Print and shaded views of the part. All mm, measured from the part's lowest x, y and z. A direction names the side the tool comes from. Give positions to 0.01 mm unless a question says otherwise; leave off trailing zeros. Loops run counter-clockwise (first coordinate to the right, second up) from the corner with the lowest first, then second, coordinate; pieces in that order, holes last. Notation, with made-up numbers: M 29,-16 L 52,-16 A33 ccw 52,18 Z; hole C -18,56 d1. An arc over 180 degrees is marked long. Answer in a Markdown table with one row per item.
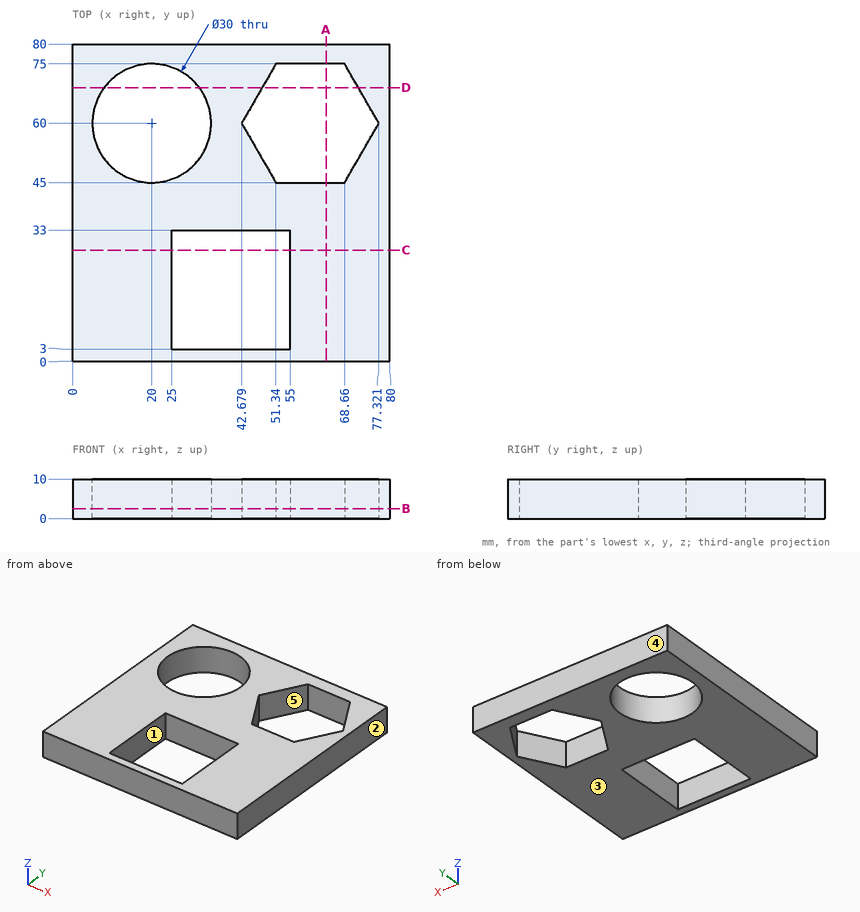
(1) Saw through at C-C, the plane y = 28. Give the cut face in (x, z), and give its area (3 significant figures).
Established:
| item | result |
|---|---|
| outline | M 0,0 L 25,0 L 25,10 L 0,10 Z; M 55,0 L 80,0 L 80,10 L 55,10 Z |
| area | 500 mm2 |
(2) Which spindle directions (+Z, -Z, +X, -X, +Y, -Y) get a long thin tool onto all of the face, cutting with end or side? Do the marked faces 4 and 5. Say none if no direction does.
Established:
| item | result |
|---|---|
| face 4 | +Z, -Z, +X, -X, +Y |
| face 5 | +Z, -Z |
(3) Mould opens along X. For the marked faces 1, 2 and 3 say: pulls with the +X half, pulls with the -X half, needs draft (parallel to the pull), parting line crosses it, or undercut.
Established:
| item | result |
|---|---|
| face 1 | undercut |
| face 2 | pulls with the +X half |
| face 3 | needs draft |
(4) Saw through at A-A, the plane x = 64. Give the cut face in (y, z).
Established:
| item | result |
|---|---|
| outline | M 0,0 L 45,0 L 45,10 L 0,10 Z; M 75,0 L 80,0 L 80,10 L 75,10 Z |
(5) Saw through at B-B, the plane z = 2.5. Give the cut face in (x, y), and give its area (3 significant figures).
Established:
| item | result |
|---|---|
| outline | M 0,0 L 80,0 L 80,80 L 0,80 Z; hole C 20,60 d30; hole M 25,3 L 55,3 L 55,33 L 25,33 Z; hole M 42.68,60 L 51.34,45 L 68.66,45 L 77.32,60 L 68.66,75 L 51.34,75 Z |
| area | 4,010 mm2 |
(6) Saw through at D-D, the plane y = 69. Give the cut face in (x, z) (1 decimal).
Established:
| item | result |
|---|---|
| outline | M 0,0 L 8,0 L 8,10 L 0,10 Z; M 32,0 L 47.9,0 L 47.9,10 L 32,10 Z; M 72.1,0 L 80,0 L 80,10 L 72.1,10 Z |
(7) Wall check: L1, parallel to X at y = 21, z = 4.25; L2, parallel to Y at x = 20, z = 8; L3, parallel to X at y = 73.5, z = 2.75 (1 decimal). Give the ranges that are in metal, low to high.
Established:
| item | result |
|---|---|
| L1 | x = 0 to 25, 55 to 80 |
| L2 | y = 0 to 45, 75 to 80 |
| L3 | x = 0 to 13.5, 26.5 to 50.5, 69.5 to 80 |
